from build123d import *

# Parameters (mm, degrees)
EXTRUDE_1_DEPTH     = 8
FILLET_1_R          = 8
FILLET_2_R          = 4
FILLET_3_R          = 4
CUT_EXTRUDE_1_DEPTH = 9
SKETCH_3_R          = 4
EXTRUDE_2_DEPTH     = 5
SKETCH_4_R          = 4
EXTRUDE_3_DEPTH     = 5


with BuildPart() as part:
    # 草图1 → 凸台-拉伸1 (new body)
    with BuildSketch(Plane(origin=(0, 0, 0), x_dir=(1, 0, 0), z_dir=(0, 1, 0))):
        Polygon((0, -130), (-75.055534995, 0), (0, 130), (75.055534995, 0), align=None)
        Polygon((57.735026919, 0), (0, -100), (-57.735026919, 0), (0, 100), align=None, mode=Mode.SUBTRACT)
    extrude(amount=EXTRUDE_1_DEPTH)

    # 圆角1
    fillet_1_edges = [part.edges().sort_by_distance(p)[0] for p in [
        (0, 4, -130),
        (0, 4, 130),
    ]]
    fillet(fillet_1_edges, radius=FILLET_1_R)

    # 圆角2
    fillet_2_edges = [part.edges().sort_by_distance(p)[0] for p in [
        (0, 4, -100),
        (0, 4, 100),
    ]]
    fillet(fillet_2_edges, radius=FILLET_2_R)

    # 圆角3
    fillet_3_edges = [part.edges().sort_by_distance(p)[0] for p in [
        (57.735026919, 4, 0),
        (-57.735026919, 4, 0),
        (75.055534995, 4, 0),
        (-75.055534995, 4, 0),
    ]]
    fillet(fillet_3_edges, radius=FILLET_3_R)

    # 草图2 → 切除-拉伸1 (cut, through all)
    with BuildSketch(Plane(origin=(0, 8, 0), x_dir=(1, 0, 0), z_dir=(0, 1, 0))):
        with BuildLine():
            Line((-9.243452109, -104.989871311), (-54.277652929, -26.988347411))
            ThreePointArc((-54.277652929, -26.988347411), (-53.179576718, -22.8902712), (-49.081500506, -23.988347411))
            Line((-49.081500506, -23.988347411), (-4.047299686, -101.989871311))
            ThreePointArc((-4.047299686, -101.989871311), (-5.145375897, -106.087947522), (-9.243452109, -104.989871311))
        make_face()
        with BuildLine():
            Line((9.243452109, -104.989871311), (54.277652929, -26.988347411))
            ThreePointArc((54.277652929, -26.988347411), (53.179576718, -22.8902712), (49.081500506, -23.988347411))
            Line((49.081500506, -23.988347411), (4.047299686, -101.989871311))
            ThreePointArc((4.047299686, -101.989871311), (5.145375897, -106.087947522), (9.243452109, -104.989871311))
        make_face()
        with BuildLine():
            Line((9.243452109, 104.989871311), (54.277652929, 26.988347411))
            ThreePointArc((54.277652929, 26.988347411), (53.179576718, 22.8902712), (49.081500506, 23.988347411))
            Line((49.081500506, 23.988347411), (4.047299686, 101.989871311))
            ThreePointArc((4.047299686, 101.989871311), (5.145375897, 106.087947522), (9.243452109, 104.989871311))
        make_face()
        with BuildLine():
            Line((-9.243452109, 104.989871311), (-54.277652929, 26.988347411))
            ThreePointArc((-54.277652929, 26.988347411), (-53.179576718, 22.8902712), (-49.081500506, 23.988347411))
            Line((-49.081500506, 23.988347411), (-4.047299686, 101.989871311))
            ThreePointArc((-4.047299686, 101.989871311), (-5.145375897, 106.087947522), (-9.243452109, 104.989871311))
        make_face()
    extrude(amount=-CUT_EXTRUDE_1_DEPTH, mode=Mode.SUBTRACT)

    # 草图3 → 凸台-拉伸2 (add)
    with BuildSketch(Plane(origin=(0, 8, 0), x_dir=(1, 0, 0), z_dir=(0, 1, 0))):
        with Locations((0, -114)):
            Circle(SKETCH_3_R)
    extrude(amount=EXTRUDE_2_DEPTH)

    # 草图4 → 凸台-拉伸3 (add)
    with BuildSketch(Plane.XZ):
        with Locations((0, -114)):
            Circle(SKETCH_4_R)
    extrude(amount=EXTRUDE_3_DEPTH)


solid = part.part
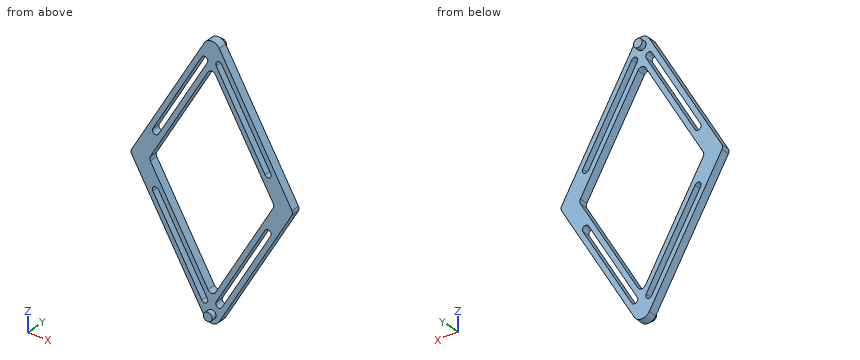
Work out the finished part from the listing and answer in its coordinate system (mm). Coordinates: 2 decimals unless noted, no trailing zeros. Write each loop counter-clockwise with the first axis right and the second up, starting at its lowest first coordinate (ties: lowest second). Pieces come first, ordered by that corner, then holes. Notation, with made-up numbers: M 60.5,8.5 L 101.5,8.5 A21 cw 101.5,15.5 Z; hole C 10,63.25 d3. An arc over 180 degrees is marked long. Write item = value, one per line.
1. The part is cut by section A-A (x = 0). Determine the outline of the cut face in (y, z), then the cut area to 3 significant figures.
Solution:
outline = M -5,-118 L 0,-118 L 0,-122 L 8,-122 L 8,-96 L 0,-96 L 0,-110 L -5,-110 Z; M 0,96 L 8,96 L 8,110 L 13,110 L 13,118 L 8,118 L 8,122 L 0,122 Z
area = 496 mm2
2. The part is cut by section C-C (y = 4). State how many separate pieces and enclosed holes the cut face has, then the cut area to 3 significant figures.
Solution:
separate_pieces = 1
enclosed_holes = 5
area = 5,630 mm2
3. The part is cut by section B-B (z = 20). Determine the outline of the cut face in (x, y), then the cut area to 3 significant figures.
Solution:
outline = M -63.51,0 L -46.19,0 L -46.19,8 L -63.51,8 Z; M 46.19,0 L 63.51,0 L 63.51,8 L 46.19,8 Z
area = 277 mm2
4. Flat-ended cylindrical pins translate along their axes: pin 1 (3 mm diameter, centred on x = 29.5, y = 5.5, fed in from -Z); pin 2 (1 mm diameter, centred on y = -1, z = 5, fed in from +X); pin 3 (5 mm diameter, centred on y = 1.5, z = 22, fed in from -X); pin 4 (2 mm diameter, centred on y = 6.5, z = -83, fed in from +X). Find the tip coordinate at first contact, or state that the pin passes through.
Solution:
pin_1 = -81.5
pin_2 = through
pin_3 = -63.8
pin_4 = 27.71
5. The part is cut by section D-D (x = -18.5). Determine the outline of the cut face in (y, z).
Solution:
outline = M 0,-97.96 L 8,-97.96 L 8,-88.96 L 0,-88.96 Z; M 0,-76.96 L 8,-76.96 L 8,-67.96 L 0,-67.96 Z; M 0,67.96 L 8,67.96 L 8,76.96 L 0,76.96 Z; M 0,88.96 L 8,88.96 L 8,97.96 L 0,97.96 Z
6. Straight lines are drawn through the part: line 1 (X direction, y = 0.25, z = 73.5); line 2 (X direction, y = 7, z = -44); line 3 (Z direction, x = -20.5, y = 3.5). For each, find the intervals that lie inside material, in ascending order. Write a range as from..to.
Solution:
line_1 = -32.62..-27.42, -20.5..-15.3, 15.3..20.5, 27.42..32.62
line_2 = -49.65..-44.46, -37.53..-32.33, 32.33..37.53, 44.46..49.65
line_3 = -94.49..-85.49, -73.49..-64.49, 64.49..73.49, 85.49..94.49
